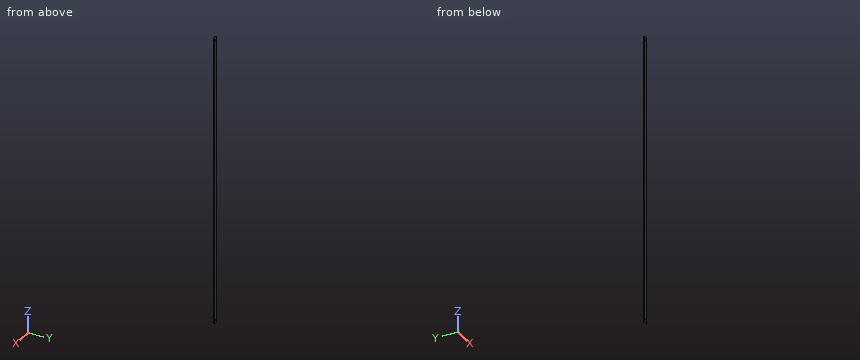
```python
from build123d import *

# Parameters (mm, degrees)
Y_KSEKLIK_EKSTR_ZYON1_DEPTH = 1800
IZIM2_R                     = 2.5
KES_EKSTR_ZYON5_DEPTH       = 10


with BuildPart() as part:
    # Çizim1 → Yükseklik-Ekstrüzyon1 (new body)
    with BuildSketch(Plane.XY):
        Polygon((0, 0), (20, 0), (15, -5), (20, -10), (0, -10), (5, -5), align=None)
    extrude(amount=Y_KSEKLIK_EKSTR_ZYON1_DEPTH)

    # Çizim2 → Kes-Ekstrüzyon5 (cut)
    with BuildSketch(Plane(origin=(0, 0, 0), x_dir=(1, 0, 0), z_dir=(0, 1, 0))):
        with Locations((10, -20)):
            Circle(IZIM2_R)
        with Locations((10, -1780)):
            Circle(IZIM2_R)
    extrude(amount=-KES_EKSTR_ZYON5_DEPTH, mode=Mode.SUBTRACT)


solid = part.part
```
Verification items for the finished model (mm, model axes). Give positions to 0.01 mm unless a question says otherwise; leave off trailing zeros. Loops run counter-clockwise (first coordinate to the right, second up) from the corner with the lowest first, then second, coordinate; pieces in that order, holes last.
1. Section check A-A, the plane y = -2. Enter the section's corners in (x, z), then the cut area to 3 significant figures.
2. Section check B-B, the plane z = 1261. Enter the section's corners in (x, y).
3. Go/stop test with flat-tipped pins: pin 1 Ø3 at (x, z) = (10, 20) entering from +Y; pin 2 Ø2 at (y, z) = (-8.5, 1030) entering from +X. Record where each tip stops, or that it passes through.
4. Thickness scan on line 1 (Z direction, x = 10, y = -4.5); line 2 (Z direction, x = 10.75, y = -1.75); line 3 (X direction, y = -4.75, z = 1780). Record the ranges inside material, lowest first.
Geometry says:
1. outline: (2, 0) - (18, 0) - (18, 1800) - (2, 1800) - close; hole circle Ø5 at (10, 20); hole circle Ø5 at (10, 1780)
1. area: 28,800 mm2
2. outline: (0, -10) - (20, -10) - (15, -5) - (20, 0) - (0, 0) - (5, -5) - close
3. pin 1: passes through
3. pin 2: stops at x = 19.5
4. line 1: z = 0 to 17.5, 22.5 to 1777.5, 1782.5 to 1800
4. line 2: z = 0 to 17.62, 22.38 to 1777.62, 1782.38 to 1800
4. line 3: x = 4.75 to 7.5, 12.5 to 15.25
